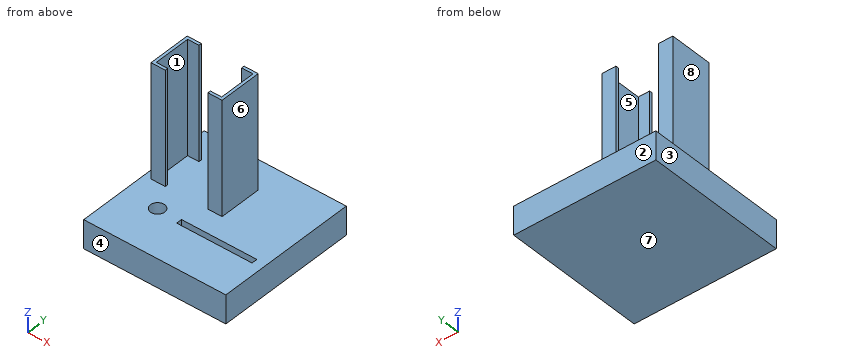
from build123d import *

# Parameters (mm, degrees)
BOX_W          = 100
BOX_H          = 100
BOX_DEPTH      = 20
CYLINDER_R     = 5
CYLINDER_DEPTH = 15
BOX001_W       = 50
BOX001_H       = 30
BOX001_DEPTH   = 80
BOX002_W       = 46
BOX002_H       = 26
BOX002_DEPTH   = 80
BOX003_W       = 30
BOX003_H       = 30
BOX003_DEPTH   = 80
BOX004_W       = 53
BOX004_H       = 4
BOX004_DEPTH   = 15


with BuildPart() as part:
    # Box → Box (join)
    with BuildSketch(Plane.XY):
        with Locations((50, 50)):
            Rectangle(BOX_W, BOX_H)
    extrude(amount=BOX_DEPTH)

    # Cylinder → Cylinder (cut)
    with BuildSketch(Plane(origin=(24, 33, 5), x_dir=(1, 0, 0), z_dir=(0, 0, 1))):
        Circle(CYLINDER_R)
    extrude(amount=CYLINDER_DEPTH, mode=Mode.SUBTRACT)

    # Box001 → Box001 (join)
    with BuildSketch(Plane(origin=(5, 50, 20), x_dir=(1, 0, 0), z_dir=(0, 0, 1))):
        with Locations((25, 15)):
            Rectangle(BOX001_W, BOX001_H)
    extrude(amount=BOX001_DEPTH)

    # Box002 → Box002 (cut)
    with BuildSketch(Plane(origin=(7, 52, 20), x_dir=(1, 0, 0), z_dir=(0, 0, 1))):
        with Locations((23, 13)):
            Rectangle(BOX002_W, BOX002_H)
    extrude(amount=BOX002_DEPTH, mode=Mode.SUBTRACT)

    # Box003 → Box003 (cut)
    with BuildSketch(Plane(origin=(15, 50, 20), x_dir=(1, 0, 0), z_dir=(0, 0, 1))):
        with Locations((15, 15)):
            Rectangle(BOX003_W, BOX003_H)
    extrude(amount=BOX003_DEPTH, mode=Mode.SUBTRACT)

    # Box004 → Box004 (cut)
    with BuildSketch(Plane(origin=(40, 30, 5), x_dir=(1, 0, 0), z_dir=(0, 0, 1))):
        with Locations((26.5, 2)):
            Rectangle(BOX004_W, BOX004_H)
    extrude(amount=BOX004_DEPTH, mode=Mode.SUBTRACT)


solid = part.part
CAD build for the part. Positions are in the model's coordinates, mm. Face numbers are marked on the shaded views. A direction names the side the tool comes from. Give positions to 0.01 mm unless a question says otherwise; leave off trailing zeros. Order: outer loops, then holes, each group sorted by start corner. A loop starts at its lowest first (then second) coordinate and runs counter-clockwise, first axis right, second up. Notation, with made-up numbers: (75, 40.25) -> (106, 40.25) arc R14 ccw to (106, 47.25) -> close; hole circle Ø7 at (-29, 64.25). An arc over 180 degrees is marked (long way). Return JSON: item names as keys, results as strings.
Q1. Flat gauge pins, fed straight in: pin 1 (10 mm diameter, centred on x = 82.5, y = 51, fed in from -Z); pin 2 (3 mm diameter, centred on x = 26.5, y = 31.5, fed in from +Z); pin 3 (24 mm diameter, centred on y = 62.5, z = 59.5, fed in from +X); pin 4 (11 mm diameter, centred on x = 12, z = 58.5, fed in from -Y). Where does each tip first touch, or does it go through?
Working result:
{"pin 1": "z = 0", "pin 2": "z = 5", "pin 3": "x = 55", "pin 4": "y = 50"}
Q2. Mould opens along X. For the marked faces 1, 2 and 3 say: pulls with the +X half, pulls with the -X half, needs draft (parallel to the pull), parting line crosses it, or undercut.
Working result:
{"face 1": "undercut", "face 2": "needs draft", "face 3": "pulls with the -X half"}
Q3. Saw through at A-A (z = 45.5). Write the cut outline in (x, y), then the cut area to 3 significant figures.
Working result:
{"outline": "(5, 50) -> (15, 50) -> (15, 52) -> (7, 52) -> (7, 78) -> (15, 78) -> (15, 80) -> (5, 80) -> close; (45, 50) -> (55, 50) -> (55, 80) -> (45, 80) -> (45, 78) -> (53, 78) -> (53, 52) -> (45, 52) -> close", "area": "184 mm²"}
Q4. Saw through at C-C (x = 24). Write the cut outline in (y, z).
Working result:
{"outline": "(0, 0) -> (100, 0) -> (100, 20) -> (38, 20) -> (38, 5) -> (28, 5) -> (28, 20) -> (0, 20) -> close"}
Q5. Saw through at B-B (y = 72.5). Write the cut outline in (x, z).
Working result:
{"outline": "(0, 0) -> (100, 0) -> (100, 20) -> (55, 20) -> (55, 100) -> (53, 100) -> (53, 20) -> (7, 20) -> (7, 100) -> (5, 100) -> (5, 20) -> (0, 20) -> close"}
Q6. Drill centre lines: line 1 (X direction, y = 75, z = 44.5); line 2 (Z direction, x = 95, y = 15.5). Where is each one in solid material? Low to high.
Working result:
{"line 1": "5 to 7, 53 to 55", "line 2": "0 to 20"}
Q7. Which spindle directions (+Z, -Z, +X, -X, +Y, -Y) get a long thin tool onto all of the face, cutting with end or side? Do the marked faces 4, 5, 6, 7 and 8. Say none if no direction does.
Working result:
{"face 4": "+Z, -Z, +X, -X, -Y", "face 5": "+Z", "face 6": "+Z, +X, +Y, -Y", "face 7": "-Z, +X, -X, +Y, -Y", "face 8": "+Z, -X, +Y, -Y"}
Q8. Saw through at D-D (y = 41.5). Write the cut outline in (x, z).
Working result:
{"outline": "(0, 0) -> (100, 0) -> (100, 20) -> (0, 20) -> close"}
